Geometry: final body of the model. Coordinates: model frame, mm. Coordinates: 2 decimals unless noted, no trailing zeros. Write each loop counter-clockwise with the first axis right and the second up, starting at its lowest first coordinate (ties: lowest second). Pieces come first, ordered by that corner, then holes.
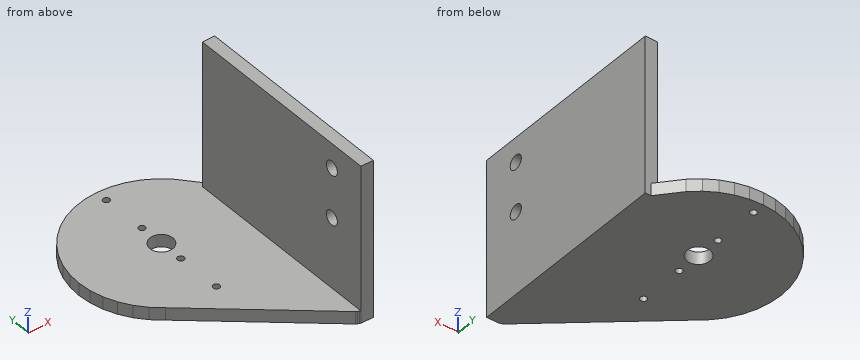
from build123d import *

# Parameters (mm, degrees)
BOSS_EXTRUDE1_START     = -26
BOSS_EXTRUDE1_DEPTH     = 3
BOSS_EXTRUDE2_START     = -26
SKETCH2_W               = 3
SKETCH2_H               = 49
BOSS_EXTRUDE2_DEPTH     = 38
CUT_EXTRUDE1_DEPTH      = 52.730068626
CUT_EXTRUDE1_DEPTH_BACK = 52.730068626
SKETCH3_R               = 2.75
SKETCH3_R_2             = 0.8
CUT_EXTRUDE2_DEPTH      = 52.730068626
CUT_EXTRUDE2_DEPTH_BACK = 52.730068626
SKETCH4_R               = 1.725


with BuildPart() as part:
    # Sketch1 → Boss-Extrude1 (new body)
    with BuildSketch(Plane.XY.offset(BOSS_EXTRUDE1_START)):
        Polygon((-20, 0), (-19.7538, -3.1287), (-19.0211, -6.1803), (-17.8201, -9.0798), (-16.1803, -11.7557), (-14.1421, -14.1421), (-11.7557, -16.1803), (16.0305, -39.5225), (16.365, -39.7275), (16.7275, -39.8776), (17.1089, -39.9692), (17.5, -40), (17.8911, -39.9692), (18.2725, -39.8776), (18.635, -39.7275), (18.9695, -39.5225), (19.2678, -39.2678), (19.5225, -38.9695), (19.7275, -38.635), (19.8776, -38.2725), (19.9692, -37.8911), (20, -37.5), (20, 6.5), (19.9692, 6.8911), (19.8776, 7.2725), (19.7275, 7.635), (19.5225, 7.9695), (19.2678, 8.2678), (14.1421, 14.1421), (11.7557, 16.1803), (9.0798, 17.8201), (6.1803, 19.0211), (3.1287, 19.7538), (0, 20), (-3.1287, 19.7538), (-6.1803, 19.0211), (-9.0798, 17.8201), (-11.7557, 16.1803), (-14.1421, 14.1421), (-16.1803, 11.7557), (-17.8201, 9.0798), (-19.0211, 6.1803), (-19.7538, 3.1287), align=None)
    extrude(amount=BOSS_EXTRUDE1_DEPTH)

    # Sketch2 → Boss-Extrude2 (add)
    with BuildSketch(Plane.XY.offset(BOSS_EXTRUDE2_START)):
        with Locations((18.5, -15.5)):
            Rectangle(SKETCH2_W, SKETCH2_H)
    extrude(amount=BOSS_EXTRUDE2_DEPTH)

    # Sketch3 → Cut-Extrude1 (cut, two sides: drawn at the far end of the back side and taken through both)
    with BuildSketch(Plane.XY.offset(-CUT_EXTRUDE1_DEPTH_BACK)):
        Circle(SKETCH3_R)
        with Locations((0, 6)):
            Circle(SKETCH3_R_2)
        with Locations((0, -6)):
            Circle(SKETCH3_R_2)
        with Locations((0, 17)):
            Circle(SKETCH3_R_2)
        with Locations((0, -17)):
            Circle(SKETCH3_R_2)
    extrude(amount=CUT_EXTRUDE1_DEPTH + CUT_EXTRUDE1_DEPTH_BACK, mode=Mode.SUBTRACT)

    # Sketch4 → Cut-Extrude2 (cut, two sides: drawn at the far end of the back side and taken through both)
    with BuildSketch(Plane(origin=(0, 0, 0), x_dir=(0, 0, -1), z_dir=(1, 0, 0)).offset(-CUT_EXTRUDE2_DEPTH_BACK)):
        with Locations((-6, -31)):
            Circle(SKETCH4_R)
        with Locations((6, -31)):
            Circle(SKETCH4_R)
    extrude(amount=CUT_EXTRUDE2_DEPTH + CUT_EXTRUDE2_DEPTH_BACK, mode=Mode.SUBTRACT)


solid = part.part
Item 1: Section D-D, the plane z = 3. Output: boundary loops of the cut face in (x, y), plus the area to 3 significant figures.
Derived:
outline: (17, -40) - (20, -40) - (20, 9) - (17, 9) - close
area: 147 mm2
Item 2: Section A-A, the plane z = -6. Output: boundary loops of the cut face in (x, y) (3 decimals), plus the area to 3 significant figures.
Derived:
outline: (17, -40) - (20, -40) - (20, -32.725) - (17, -32.725) - close; (17, -29.275) - (20, -29.275) - (20, 9) - (17, 9) - close
area: 137 mm2
Item 3: Material intervals for probe 1 along Y at (x, z) = (0, -24); probe 2 along Y at (x, z) = (17.9, -6) (3 decimals); probe 3 along Z at (x, y) = (9, -8), sorted ascending.
Derived:
probe 1: y = -26.06 to -17.8, -16.2 to -6.8, -5.2 to -2.75, 2.75 to 5.2, 6.8 to 16.2, 17.8 to 20
probe 2: y = -40 to -32.725, -29.275 to 9
probe 3: z = -26 to -23
Item 4: Section B-B, the plane y = -32. Output: boundary loops of the cut face in (x, z), plus the area to 3 significant figures.
Derived:
outline: (7.08, -26) - (20, -26) - (20, -7.41) - (17, -7.41) - (17, -23) - (7.08, -23) - close; (17, -4.59) - (20, -4.59) - (20, 4.59) - (17, 4.59) - close; (17, 7.41) - (20, 7.41) - (20, 12) - (17, 12) - close
area: 127 mm2
Item 5: Pin query (flat end, axial travel): pin 1 (4 mm diameter, centred on y = 7, z = -1.5, fed in from -X); pin 2 (2.5 mm diameter, centred on x = 0, y = -6, fed in from +Z); pin 3 (1.5 mm diameter, centred on x = 18, z = -7.5, fed in from +Y). Return the tip coordinate at first contact, or that it passes through.
Derived:
pin 1: stops at x = 17
pin 2: stops at z = -23
pin 3: stops at y = 9
Item 6: Section C-C, the plane y = 17. Output: boundary loops of the cut face in (x, z).
Derived:
outline: (-10.42, -26) - (-0.8, -26) - (-0.8, -23) - (-10.42, -23) - close; (0.8, -26) - (10.42, -26) - (10.42, -23) - (0.8, -23) - close
